Source: CAD feature listing. Evaluate the final solid. Frame: model axes, mm. A direction names the side the tool comes from. Coordinates: 2 decimals unless noted, no trailing zeros. Order: outer loops, then holes, each group sorted by start corner. A loop starts at its lowest first (then second) coordinate and runs counter-clockwise, first axis right, second up.
Item 1: Section D-D on z = -8. Return the cut outline in (x, y).
Item 2: Mould query, pull axis Z, two halves, no side actions, for faces 1 (the cylindrical face through (-1.73, 7.81, -8.62)), 2 (the flat face through (0, 0, 145)), 3 (the flat face through (-5.4, -6.2, 0)), 4 (the cylindrical face through (3.398, -25.878, 43.877)). Classes: released by +Z, released by -Z, zero draft, split by the parting line, or undercut.
Item 3: Ray query, line 1 (Z direction, x = -5, y = 16); line 2 (Z direction, x = 2.5, y = 8); line 3 (Y direction, x = 16, z = 88). Return the intervals inside material, ascending.
Item 4: Contact query for flat-ended pins moving along their axis: P1, Ø3, axis at y = 3, z = 11, coming from the +X side; P2, Ø3, axis at x = 16, y = 0, coming from the +Z side; P3, Ø8, axis at x = -15, z = 62, coming from the +Y side; P4, Ø12, axis at x = 17.5, z = 111, coming from the +Y side. Output: stop coordinate, or through.
Item 5: Section C-C on z = 19. Return the cut outline in (x, y).
Item 6: Reachability of faces 5 (the flat face through (-5.4, 6.2, -17)), 6 (the cylindrical face through (11.923, 3.755, 93.451)), 7 (the flat face through (0, 0, -37)) from +Z, -Z, +X, -X, +Y, -Y: full face, straight path, thin tool, end or side. Return the list, or none.
Item 7: Section A-A on x = 0. Return the cut outline in (y, z), then the cut area to 3 significant figures.
from build123d import *

# Parameters (mm, degrees)
SKETCH_1_R          = 26.1
EXTRUDE_1_DEPTH     = 90
FILLET_1_R          = 1
SKETCH_2_R          = 12.5
EXTRUDE_2_DEPTH     = 7
SKETCH_3_R          = 8
EXTRUDE_3_DEPTH     = 48
SKETCH_4_R          = 2.5
CUT_EXTRUDE_1_DEPTH = 5
SKETCH_1_2_R        = 26.1
EXTRUDE_4_DEPTH     = 10
EXTRUDE_START       = 17
SKETCH_6_R          = 8
EXTRUDE_5_DEPTH     = 17
EXTRUDE_START_2     = 20
SKETCH_7_R          = 26.1
EXTRUDE_6_DEPTH     = 20


with BuildPart() as part:
    # Sketch 1 → Extrude 1 (new body)
    with BuildSketch(Plane.XY):
        with Locations(Location((0, 0, 0), (0, 0, 180))):
            Circle(SKETCH_1_R)
    extrude(amount=EXTRUDE_1_DEPTH)

    # Fillet 1
    fillet_1_edges = [part.edges().sort_by_distance(p)[0] for p in [
        (26.1, 0, 90),
    ]]
    fillet(fillet_1_edges, radius=FILLET_1_R)

    # Sketch 2 → Extrude 2 (add)
    with BuildSketch(Plane.XY.offset(90)):
        Circle(SKETCH_2_R)
    extrude(amount=EXTRUDE_2_DEPTH)

    # Sketch 3 → Extrude 3 (add)
    with BuildSketch(Plane.XY.offset(97)):
        Circle(SKETCH_3_R)
    extrude(amount=EXTRUDE_3_DEPTH)

    # Sketch 4 → Cut-Extrude 1 (cut)
    with BuildSketch(Plane.XY.offset(90)):
        with Locations((-16, 0)):
            Circle(SKETCH_4_R)
        with Locations((16, 0)):
            Circle(SKETCH_4_R)
    extrude(amount=-CUT_EXTRUDE_1_DEPTH, mode=Mode.SUBTRACT)

    # Sketch 1_2 → Extrude 4 (add)
    with BuildSketch(Plane.XY):
        with Locations(Location((0, 0, 0), (0, 0, 180))):
            Circle(SKETCH_1_2_R)
    extrude(amount=EXTRUDE_4_DEPTH)

    # Sketch 6 → Extrude 5 (add)
    with BuildSketch(Plane(origin=(0, 0, 0), x_dir=(-1, 0, 0), z_dir=(0, 0, -1)).offset(EXTRUDE_START)):
        with Locations(Location((0, 0, 0), (0, 0, 180))):
            Circle(SKETCH_6_R)
    extrude(amount=-EXTRUDE_5_DEPTH)

    # Sketch 7 → Extrude 6 (add)
    with BuildSketch(Plane(origin=(0, 0, -17), x_dir=(-1, 0, 0), z_dir=(0, 0, -1)).offset(EXTRUDE_START_2)):
        Circle(SKETCH_7_R)
    extrude(amount=-EXTRUDE_6_DEPTH)


solid = part.part
Answer list:
1. outline: circle Ø16 at (0, 0)
2. face 1: undercut
2. face 2: released by +Z
2. face 3: undercut
2. face 4: zero draft
3. line 1: z = -37 to -17, 0 to 90
3. line 2: z = -37 to -17, 0 to 97
3. line 3: y = -20.62 to -2.5, 2.5 to 20.62
4. P1: stops at x = 26.06
4. P2: stops at z = 85
4. P3: stops at y = 23.67
4. P4: passes through
5. outline: circle Ø52.2 at (0, 0)
6. face 5: none
6. face 6: +Z
6. face 7: -Z, +X, -X, +Y, -Y
7. outline: (-26.1, -37) - (26.1, -37) - (26.1, -17) - (8, -17) - (8, 0) - (26.1, 0) - (26.1, 89) arc R1 ccw to (25.1, 90) - (12.5, 90) - (12.5, 97) - (8, 97) - (8, 145) - (-8, 145) - (-8, 97) - (-12.5, 97) - (-12.5, 90) - (-25.1, 90) arc R1 ccw to (-26.1, 89) - (-26.1, 0) - (-8, 0) - (-8, -17) - (-26.1, -17) - close
7. area: 6,960 mm2
